from build123d import *

# Parameters (mm, degrees)
BOSS_EXTRUDE1_DEPTH                      = 3
BOSS_EXTRUDE2_START                      = 22
BOSS_EXTRUDE2_DEPTH                      = 3
SKETCH3_W                                = 1.5
SKETCH3_H                                = 28
F_3_0MM_CLEARANCE_DOWEL_HOLE1_AT_2_COUNT = 2
F_3_0MM_CLEARANCE_DOWEL_HOLE1_AT_2_PITCH = 28.1
SKETCH5_W                                = 43.073811931
SKETCH5_H                                = 3.925670489
BOSS_EXTRUDE3_DEPTH                      = 22
SKETCH6_W                                = 12.9
SKETCH6_H                                = 5.8
CUT_EXTRUDE1_DEPTH                       = 10
SKETCH7_W                                = 5.8
SKETCH7_H                                = 1
BOSS_EXTRUDE4_DEPTH                      = 2


with BuildPart() as part:
    # Sketch1 → Boss-Extrude1 (new body)
    with BuildSketch(Plane(origin=(0, 0, 0), x_dir=(1, 0, 0), z_dir=(0, 1, 0))):
        with BuildLine():
            Line((-4.577926811, 9.356292891), (42.056666031, -6.499468675))
            ThreePointArc((42.056666031, -6.499468675), (42.793295664, -7.04620955), (43.073811931, -7.919627792))
            Line((43.073811931, -7.919627792), (43.073811931, -11.845298281))
            Line((43.073811931, -11.845298281), (0, -11.845298281))
            Line((0, -11.845298281), (0, 0.154701719))
            Line((0, 0.154701719), (-36.926188069, 0.154701719))
            Line((-36.926188069, 0.154701719), (-36.926188069, 10.154701719))
            Line((-36.926188069, 10.154701719), (-9.406467809, 10.154701719))
            ThreePointArc((-9.406467809, 10.154701719), (-6.959415254, 9.953753506), (-4.577926811, 9.356292891))
        make_face()
    extrude(amount=-BOSS_EXTRUDE1_DEPTH)


with BuildPart() as body_2:
    # Sketch1<2> → Boss-Extrude2 (new body)
    with BuildSketch(Plane(origin=(0, 0, 0), x_dir=(1, 0, 0), z_dir=(0, 1, 0)).offset(BOSS_EXTRUDE2_START)):
        with BuildLine():
            Line((-4.577926811, 9.356292891), (42.056666031, -6.499468675))
            ThreePointArc((42.056666031, -6.499468675), (42.793295664, -7.04620955), (43.073811931, -7.919627792))
            Line((43.073811931, -7.919627792), (43.073811931, -11.845298281))
            Line((43.073811931, -11.845298281), (0, -11.845298281))
            Line((0, -11.845298281), (0, 0.154701719))
            Line((0, 0.154701719), (-36.926188069, 0.154701719))
            Line((-36.926188069, 0.154701719), (-36.926188069, 10.154701719))
            Line((-36.926188069, 10.154701719), (-9.406467809, 10.154701719))
            ThreePointArc((-9.406467809, 10.154701719), (-6.959415254, 9.953753506), (-4.577926811, 9.356292891))
        make_face()
    extrude(amount=BOSS_EXTRUDE2_DEPTH)


with BuildPart() as f_3_0mm_clearance_dowel_hole1_tool:
    # Sketch3 → Ø3.0mm Clearance Dowel Hole1 (revolve)
    with BuildSketch(Plane(origin=(-33.926188069, -3, -5.154701719), x_dir=(0, 0, -1), z_dir=(1, 0, 0))):
        with Locations((0.75, 14)):
            Rectangle(SKETCH3_W, SKETCH3_H)
    f_3_0mm_clearance_dowel_hole1 = revolve(axis=Axis((-33.926188069, -9.35, -5.154701719), (0, 1, 0)))


with BuildPart() as part_1:
    add(part.part)

    # Ø3.0mm Clearance Dowel Hole1: cut by f_3_0mm_clearance_dowel_hole1_tool
    add(f_3_0mm_clearance_dowel_hole1_tool.part, mode=Mode.SUBTRACT)


with BuildPart() as body_2_1:
    add(body_2.part)

    # Ø3.0mm Clearance Dowel Hole1: cut by f_3_0mm_clearance_dowel_hole1_tool
    add(f_3_0mm_clearance_dowel_hole1_tool.part, mode=Mode.SUBTRACT)


with BuildPart() as f_3_0mm_clearance_dowel_hole1_at_2_tool:
    # Ø3.0mm Clearance Dowel Hole1 at 2: Ø3.0mm Clearance Dowel Hole1 ×2
    with Locations(*[(i * F_3_0MM_CLEARANCE_DOWEL_HOLE1_AT_2_PITCH, 0, 0) for i in range(1, F_3_0MM_CLEARANCE_DOWEL_HOLE1_AT_2_COUNT)]):
        add(f_3_0mm_clearance_dowel_hole1)


with BuildPart() as part_2:
    add(part_1.part)

    # Ø3.0mm Clearance Dowel Hole1 at 2: cut by f_3_0mm_clearance_dowel_hole1_at_2_tool
    add(f_3_0mm_clearance_dowel_hole1_at_2_tool.part, mode=Mode.SUBTRACT)



with BuildPart() as body_2_2:
    add(body_2_1.part)

    # Ø3.0mm Clearance Dowel Hole1 at 2: cut by f_3_0mm_clearance_dowel_hole1_at_2_tool
    add(f_3_0mm_clearance_dowel_hole1_at_2_tool.part, mode=Mode.SUBTRACT)


with BuildPart() as part_3:
    add(part_2.part)

    add(body_2_2.part)  # Boss-Extrude3 merges body 2
    # Sketch5 → Boss-Extrude3 (add)
    with BuildSketch(Plane(origin=(0, 0, 0), x_dir=(1, 0, 0), z_dir=(0, 1, 0))):
        with Locations((21.536905966, -9.882463037)):
            Rectangle(SKETCH5_W, SKETCH5_H)
    extrude(amount=BOSS_EXTRUDE3_DEPTH)

    # Sketch6 → Cut-Extrude1 (cut)
    with BuildSketch(Plane(origin=(0, 25, 0), x_dir=(1, 0, 0), z_dir=(0, 1, 0))):
        with Locations((19.45, -4.945298281)):
            Rectangle(SKETCH6_W, SKETCH6_H)
    extrude(amount=-CUT_EXTRUDE1_DEPTH, mode=Mode.SUBTRACT)

    # Sketch7 → Boss-Extrude4 (add)
    with BuildSketch(Plane(origin=(13, 0, 0), x_dir=(0, 0, -1), z_dir=(1, 0, 0))):
        with Locations((-4.945298281, 24.5)):
            Rectangle(SKETCH7_W, SKETCH7_H)
    extrude(amount=BOSS_EXTRUDE4_DEPTH)


solid = part_3.part
Geometry: final body of the model. Coordinates: model frame, mm. A direction names the side the tool comes from. Round coordinates to 2 decimals unless told otherwise and drop trailing zeros. Loops run counter-clockwise (first coordinate to the right, second up) from the corner with the lowest first, then second, coordinate; pieces in that order, holes last. Notation, with made-up numbers: M 28,43 L 73,43 A8 ccw 73,50 Z; hole C 16,-19.5 d7. An arc over 180 degrees is marked long. Put each result on its own line as item: value. Start each with the question number.
(1) Section query A-A (x = -28). Return loops of the section in (y, z).
(2) Section query D-D (y = 2.75). Return loops of the section in (x, z), then the cut area to 3 significant figures.
(3) Contact query for flat-ended pins moving along their axis: pin 1 Ø10 at (x, y) = (-3, 13.5) entering from +Z; pin 2 Ø2.5 at (x, y) = (16.5, 23.5) entering from -Z; pin 3 Ø2.5 at (x, y) = (-24, 23.5) entering from +Z; pin 4 Ø6 at (y, z) = (7.5, 6) entering from -X. Output: stop coordinate, or through.
(4) Section query C-C (z = 3.5). Return loops of the section in (x, y), then the cut area to 3 significant figures.
(5) Section query B-B (z = -2). Return loops of the section in (x, y).
(6) Material intervals for line 1 along Y through (x, z) = (1, 4.75); line 2 along Z through (x, y) = (24, 12.25); line 3 along X through (y, z) = (18, 8.5), sorted ascending. Write a range as [from, to].
(7) Set-up query: faces 1 (the face through (0, 11, 9)), 2 (the face through (-5, 22, -1)), 3 (the face through (25.9, 24, 5)). Return all of +Z, -Z, +X, -X, +Y, -Y with unobstructed straight access to the full face (end or side cutting, diameter ignored); none if empty.
(8) Draft query along Z for faces 4 (the face through (19, 24, 2.045)), 5 (the face through (-6.99, -1.48, -9.96)), 6 (the face through (-36.926, 23, -5)). Return one class per face: +Z half, -Z half, draft (parallel to the pull), parting line (faces both ways), or undercut.
Findings below:
1. outline: M -3,-10.15 L 0,-10.15 L 0,-0.15 L -3,-0.15 Z; M 22,-10.15 L 25,-10.15 L 25,-0.15 L 22,-0.15 Z
2. outline: M 0,7.92 L 43.07,7.92 L 43.07,11.85 L 0,11.85 Z
2. area: 169 mm2
3. pin 1: stops at z = 11.85
3. pin 2: stops at z = -2.61
3. pin 3: stops at z = -0.15
3. pin 4: stops at x = 0
4. outline: M 0,-3 L 33.23,-3 L 33.23,0 L 0,0 Z; M 0,22 L 13,22 L 13,24 L 15,24 L 15,25 L 0,25 Z; M 25.9,22 L 33.23,22 L 33.23,25 L 25.9,25 Z
4. area: 163 mm2
5. outline: M -36.93,-3 L 17.06,-3 L 17.06,0 L -36.93,0 Z; M -36.93,22 L 17.06,22 L 17.06,25 L -36.93,25 Z
6. line 1: y = [-3, 0], [22, 25]
6. line 2: z = [7.92, 11.85]
6. line 3: x = [0, 43.07]
7. face 1: +Z, -X, +Y, -Y
7. face 2: -Z, +X, -X
7. face 3: +Y
8. face 4: undercut
8. face 5: -Z half
8. face 6: draft
